from build123d import *

# Parameters (mm, degrees)
F0_W     = 70
F0_H     = 28.9502215247
F1_DEPTH = 17.5
F3_DEPTH = 70.001
F5_DEPTH = 70.001
F6_SCALE = 1.5


with BuildPart() as f1:
    # F0 (on Top) → F1 (new body)
    with BuildSketch(Plane.XY):
        with Locations((-18.1001285091, -2.3733787239)):
            Rectangle(F0_W, F0_H)
    extrude(amount=F1_DEPTH)

    # F2 (on face) → F3 (cut, through all)
    with BuildSketch(Plane.YZ.offset(16.8998714909)):
        Polygon((-16.8484894862, 17.5), (-16.8484894862, 1.9115059404), (10.3485193104, 17.5), align=None)
        Polygon((12.1017320385, 15.7691705972), (-15.4105003687, 0), (12.1017320385, 0), align=None)
    extrude(amount=-F3_DEPTH, mode=Mode.SUBTRACT)

    # F4 (on face) → F5 (cut, through all)
    with BuildSketch(Plane.YZ.offset(16.8998714909)):
        Polygon((10.3485193104, 17.5), (6.6982309879, 15.4077663189), (6.6982309879, 12.6720489741), (12.1017320385, 15.7691705972), (12.1017320385, 17.5), align=None)
    extrude(amount=-F5_DEPTH, mode=Mode.SUBTRACT)


with BuildPart() as f1_1:
    # F6: moved
    add(f1.part.scale(F6_SCALE).moved(Location((-8.4499357454, 8.4242447431, -0.9557529702))))


solid = f1_1.part
The listing builds one solid part. Answer for the finished solid, in the listing's coordinates (mm). Round coordinates to 2 decimals unless told otherwise and drop trailing zeros. Write each loop counter-clockwise with the first axis right and the second up, starting at its lowest first coordinate (ties: lowest second). Pieces come first, ordered by that corner, then holes. Notation, with made-up numbers: (19.5, 19) - (74.5, 19) arc R22 ccw to (74.5, 53) - close; hole circle Ø1 at (61.25, 2). An arc over 180 degrees is marked (long way). Use a Markdown table: item, result. Add a question column.
1. The part is cut by section C-C (z = 0.5). Write down the section's boundary in (x, y), and give its area (3 significant figures).
2. The part is cut by section A-A (x = -20.5). Write down the section's boundary in (y, z).
3. Consider line 1 (Z direction, x = -61, y = -5.5); line 2 (Z direction, x = -75, y = -10); line 3 (Y direction, x = -68.5, z = 13). Determine where each line is inside the solid, lowest interval first.
4. Flat-ended cylindrical pins translate along their axes: P1, Ø2, axis at x = -70, y = 0, coming from the +Z side; P2, Ø4, axis at x = -13.5, z = 4, coming from the -Y side; P3, Ø12, axis at x = -51, z = 6, coming from the +Y side; P4, Ø1.5, axis at y = 13, z = 12.5, coming from the -X side. Find the tip coordinate at first contact, or state that the pin passes through.
5. The part is cut by section B-B (y = -0.5). Write down the section's boundary in (x, z), and give its area (3 significant figures).
Reported:
| question | item | result |
|---|---|---|
| 1 | outline | (-88.1, -16.85) - (16.9, -16.85) - (16.9, -12.15) - (-88.1, -12.15) - close |
| 1 | area | 493 mm^2 |
| 2 | outline | (-16.85, -0.96) - (-14.69, -0.96) - (18.47, 18.05) - (18.47, 22.16) - (-16.85, 1.91) - close |
| 3 | line 1 | 4.31 to 8.42 |
| 3 | line 2 | 1.73 to 5.84 |
| 3 | line 3 | 2.5 to 9.66 |
| 4 | P1 | z = 12.14 |
| 4 | P2 | y = -16.69 |
| 4 | P3 | y = 7.91 |
| 4 | P4 | through |
| 5 | outline | (-88.1, 7.18) - (16.9, 7.18) - (16.9, 11.28) - (-88.1, 11.28) - close |
| 5 | area | 431 mm^2 |
